Geometry: final body of the model. Coordinates: model frame, mm. Give positions to 0.01 mm unless a question says otherwise; leave off trailing zeros. Loops run counter-clockwise (first coordinate to the right, second up) from the corner with the lowest first, then second, coordinate; pieces in that order, holes last.
1. Material intervals for line 1 along Y through (x, z) = (-1733, 13); line 2 along X through (y, z) = (-502, 14.75); line 3 along X through (y, z) = (-1168.5, 9.5), sorted ascending.
2. Section A-A, the plane z = 7.25. Output: boundary loops of the cut face in (x, y), then the cut area to 3 significant figures.
3. Section B-B, the plane y = -1110. Output: boundary loops of the cut face in (x, z), then the cut area to 3 significant figures.
4. Section C-C, the plane x = -820. Output: boundary loops of the cut face in (y, z), then the cut area to 3 significant figures.
5. First-contact query: P1, Ø6.5, axis at y = -947.5, z = 7.5, coming from the -X side; P2, Ø10, axis at x = -1162, z = 7.5, coming from the -Y side; P3, Ø4, axis at x = -595, z = 12, coming from the -Y side. Flat tips, straight axial feed; report the tip coordinate or a pass-through.
from build123d import *

# Parameters (mm, degrees)
F1_DEPTH = 19.05
F2_R     = 12.7
F3_R     = 6.35
F4_R     = 6.35


with BuildPart() as f1:
    # F0 (on Top) → F1 (new body)
    with BuildSketch(Plane.XY):
        Polygon((0, -1219.2), (0, 0), (-2514.6, 0), (-2514.6, -508), (-660.4, -508), (-457.2, -711.2), (-457.2, -1219.2), align=None)
    extrude(amount=F1_DEPTH)

    # F2
    f2_edges = [f1.edges().sort_by_distance(p)[0] for p in [
        (-660.4, -508, 9.525),
        (-457.2, -711.2, 9.525),
    ]]
    fillet(f2_edges, radius=F2_R)

    # F3
    f3_edges = [f1.edges().sort_by_distance(p)[0] for p in [
        (-1590.130256, -508, 19.05),
    ]]
    fillet(f3_edges, radius=F3_R)

    # F4
    f4_edges = [f1.edges().sort_by_distance(p)[0] for p in [
        (-225.425, -1219.2, 19.05),
        (-2514.6, -250.825, 19.05),
    ]]
    fillet(f4_edges, radius=F4_R)


solid = f1.part
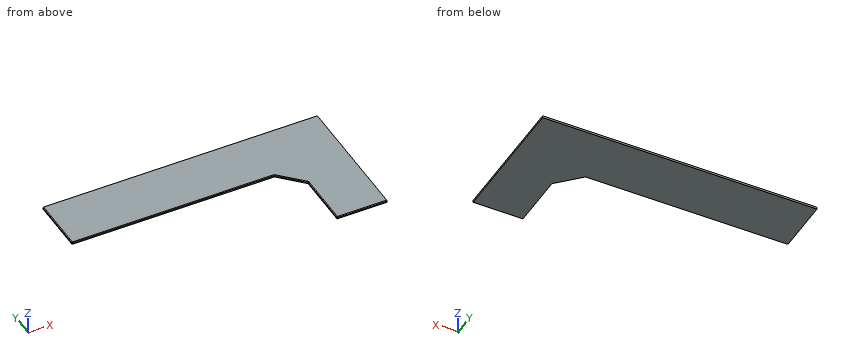
Answers below:
1. line 1: y = -507.99 to 0
1. line 2: x = -2514.25 to 0
1. line 3: x = -457.2 to 0
2. outline: (-2514.6, -501.65) arc R6.35 ccw to (-2508.25, -508) - (-665.66, -508) arc R12.7 cw to (-656.68, -511.72) - (-460.92, -707.48) arc R12.7 cw to (-457.2, -716.46) - (-457.2, -1212.85) arc R6.35 ccw to (-450.85, -1219.2) - (0, -1219.2) - (0, 0) - (-2514.6, 0) - close
2. area: 1,620,000 mm2
3. outline: (-457.2, 0) - (0, 0) - (0, 19.05) - (-450.85, 19.05) arc R6.35 ccw to (-457.2, 12.7) - close
3. area: 8,700 mm2
4. outline: (-508, 0) - (0, 0) - (0, 19.05) - (-501.65, 19.05) arc R6.35 ccw to (-508, 12.7) - close
4. area: 9,670 mm2
5. P1: stops at x = -457.2
5. P2: stops at y = -508
5. P3: stops at y = -575.4
